Solid Edge part; units mm, degrees
sketch "Sketch1" plane through (0, 0, 0) normal (0, 0, 1) x (1, 0, 0)
  line L0 (86.627, 26.9205) -> (86.627, 0)
  line L1 (86.627, -26.9205) -> (86.627, 0)
  line L2 (28.085, -26.9205) -> (86.627, -26.9205)
  line L3 (28.085, 26.9205) -> (86.627, 26.9205)
  arc A0 (28.085, -26.9205) -> (28.085, 26.9205) centre (0, 0) cw
extrude "Protrusion1" add sketch "Sketch1" along normal blind 7
fillet "Redondeo_1" radius 10 2 edges at (86.627, 26.9205, 3.5) (86.627, -26.9205, 3.5)
sketch "Sketch2" plane through (23.8618, 0, 7) normal (0, 0, 1) x (1, 0, 0)
  circle A0 centre (-47.8618, 0) radius 1.6
  circle A1 centre (-23.8618, 0) radius 2.5
  circle A2 centre (0.1382, 0) radius 1.6
  circle A3 centre (24.1773, 15.5) radius 2.25
  circle A4 centre (24.1773, -15.5) radius 2.25
  circle A5 centre (39.6793, 0) radius 11.24
  circle A6 centre (55.1773, -15.5) radius 2.25
  circle A7 centre (55.1773, 15.5) radius 2.25
extrude "Cutout1" cut sketch "Sketch2" against normal up to next
sketch "Sketch3" plane through (52.356, -26.9205, 3.5) normal (0, -1, 0) x (1, 0, 0)
  line L0 (34.271, -0.777) -> (-14.645, -0.777)
  line L1 (-14.645, -0.777) -> (-18.713, -3.5)
  line L2 (-18.713, -3.5) -> (34.271, -3.5)
  line L3 (34.271, -3.5) -> (34.271, -0.777)
extrude "Cutout2" cut sketch "Sketch3" against normal up to next
sketch "Sketch4" plane through (-2.6302, 0, 0) normal (0, 0, -1) x (0, 1, 0)
  arc A0 (14.1561, 36.2733) -> (-14.1561, 36.2733) centre (0, 2.6302) cw construction
  circle A1 centre (0, 2.6302) radius 36.5
  circle A2 centre (0, 2.6302) radius 27.5
extrude "VaciadoExtruido_3" cut sketch "Sketch4" against normal blind 2.5
Part model, mm, in its own coordinate system. A direction names the side the tool comes from. Coordinates: 2 decimals unless noted, no trailing zeros. Order: outer loops, then holes, each group sorted by start corner. A loop starts at its lowest first (then second) coordinate and runs counter-clockwise, first axis right, second up. Notation, with made-up numbers: (-6, 12) - (21, 12) arc R13 cw to (21, 33) - close; hole circle Ø8 at (49.5, 47). An arc over 180 degrees is marked (long way). Return JSON: item names as keys, results as strings. Group by question number.
Item 1: Cut at D-D (y = -15.5). List the corners of the cut face in (x, z), plus the area to 3 significant figures.
Item 2: Pin check, flat tips, straight feed: pin 1 (2 mm diameter, centred on x = 41, z = 6, fed in from -Y); pin 2 (4 mm diameter, centred on x = 66.5, y = 15, fed in from -Z); pin 3 (3.5 mm diameter, centred on x = 45, z = 3, fed in from +Y). Stop position of each tip, or through.
Item 3: Drill centre lines: probe 1 along Y at (x, z) = (24, 1.75); probe 2 along Z at (x, y) = (63, -14.5); probe 3 along X at (y, z) = (25, 2.25). Where is each one in solid material? Low to high. Write a range as from..to.
Item 4: Pull direction Y, two halves, no side cores. Call faces 4 (the face through (37.061, -0.377, 2.288)), 5 (the face through (49.077, 13.504, 4.891)), 6 (the face through (-38.882, -1.295, 3.451)), 7 (the face through (52, 26.92, 5)): pulls with the +Y half, pulls with the -Y half, needs draft (parallel to the pull), parting line crosses it, or undercut.
Item 5: Which spindle directions (+Z, -Z, +X, -X, +Y, -Y) get a long thin tool onto all of the face, cutting with end or side? Do faces 1 (the face through (52, 0, 2.723)), 2 (the face through (-35.632, -7.912, 1.232)), 3 (the face through (52, -26.92, 5)). Say none if no direction does.
Item 6: Cut at B-B (z = 5.75). State how many separate pieces and enclosed holes the cut face has, plus the area to 3 significant figures.
Item 7: Cut at A-A (x = 0). List the corners of the cut face in (y, z), plus the area to 3 significant figures.
Item 8: Cut at C-C (y = 5.5). List the corners of the cut face in (x, z), plus the area to 3 significant figures.
Check values:
{
 "1": {"outline": "(-35.68, 0) - (-33.05, 0) - (-33.05, 2.5) - (-22.72, 2.5) - (-22.72, 0) - (22.72, 0) - (22.72, 2.5) - (33.05, 2.5) - (33.05, 0) - (33.64, 0) - (37.71, 2.72) - (45.79, 2.72) - (45.79, 7) - (-35.68, 7) - close; (50.29, 2.72) - (76.79, 2.72) - (76.79, 7) - (50.29, 7) - close; (81.29, 2.72) - (86.63, 2.72) - (86.63, 7) - (81.29, 7) - close", "area": "627 mm2"},
 "2": {"pin 1": "stops at y = -26.92", "pin 2": "stops at z = 2.72", "pin 3": "stops at y = 26.92"},
 "3": {"probe 1": "y = -30.62..-27.5, -13.43..-1.6, 1.6..13.43, 27.5..30.62", "probe 2": "z = 2.72..7", "probe 3": "x = -29.81..-26.59, -11.46..11.46, 26.59..37"},
 "4": {"face 4": "needs draft", "face 5": "undercut", "face 6": "parting line crosses it", "face 7": "pulls with the +Y half"},
 "5": {"face 1": "-Z, +X, +Y, -Y", "face 2": "-Z", "face 3": "+Z, -Z, +X, -Y"},
 "6": {"separate pieces": "1", "enclosed holes": "8", "area": "6,970 mm2"},
 "7": {"outline": "(-38.9, 0) - (-36.5, 0) - (-36.5, 2.5) - (-27.5, 2.5) - (-27.5, 0) - (-2.5, 0) - (-2.5, 7) - (-38.9, 7) - close; (2.5, 0) - (27.5, 0) - (27.5, 2.5) - (36.5, 2.5) - (36.5, 0) - (38.9, 0) - (38.9, 7) - (2.5, 7) - close", "area": "465 mm2"},
 "8": {"outline": "(-38.51, 0) - (-36.08, 0) - (-36.08, 2.5) - (-26.94, 2.5) - (-26.94, 0) - (26.94, 0) - (26.94, 2.5) - (36.08, 2.5) - (36.08, 1.63) - (37.71, 2.72) - (53.74, 2.72) - (53.74, 7) - (-38.51, 7) - close; (73.34, 2.72) - (86.63, 2.72) - (86.63, 7) - (73.34, 7) - close", "area": "610 mm2"}
}
